Build history of the part. All positions in model axes, mm. Round coordinates to 2 decimals unless told otherwise and drop trailing zeros. Write each loop counter-clockwise with the first axis right and the second up, starting at its lowest first coordinate (ties: lowest second). Pieces come first, ordered by that corner, then holes. Notation, with made-up numbers: (31.25, -10.5) - (47.25, -10.5) arc R25 cw to (47.25, 25.5) - close; hole circle Ø6 at (67, 70). An arc over 180 degrees is marked (long way). Write each question's results on one line, items separated by ' | '.
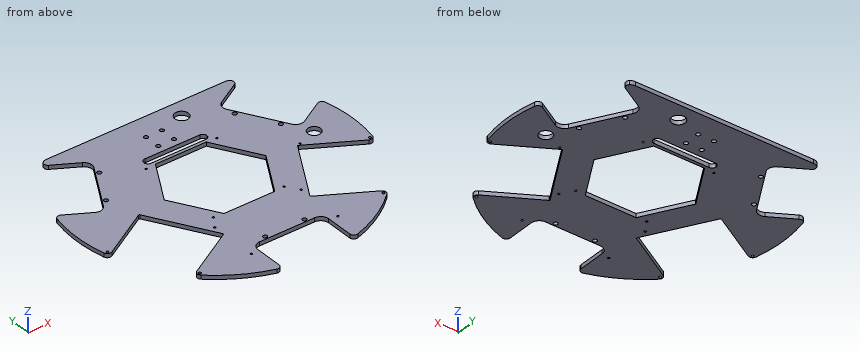
from build123d import *

# Parameters (mm, degrees)
SKETCH_1_R                   = 175
EXTRUDE_1_DEPTH              = 5
CUT_EXTRUDE_1_DEPTH          = 248.53787589
CUT_EXTRUDE_2_DEPTH          = 248.53787589
CUT_EXTRUDE_5_DEPTH          = 248.53787589
CUT_EXTRUDE_4_DEPTH          = 248.53787589
HOLE_WIZARD_M5_1_D           = 5.3
FILLET_1_R                   = 1
FILLET_2_R                   = 10
FILLET_3_R                   = 5
PATTERN_CIRCULAR_1_OUTLINE_R = 2.65
PATTERN_CIRCULAR_1_DEPTH     = 5
HOLE_WIZARD_M5_2_D           = 5.3
SKETCH_15_R                  = 8.55
CUT_EXTRUDE_3_DEPTH          = 243.280431899
MIRROR_1_DEPTH               = 5
SKETCH_18_W                  = 80
SKETCH_18_H                  = 10
CUT_EXTRUDE_6_DEPTH          = 243.280431899
FILLET_4_R                   = 5
M4X0_7_3_D                   = 3.3
SKETCH_33_R                  = 8.05
CUT_EXTRUDE_7_DEPTH          = 243.280431899
M3X0_5_2_D                   = 2.5
M3X0_5_3_D                   = 2.5
FILLET_5_R                   = 10


with BuildPart() as part:
    # 草圖1 → 填料-伸長1 (new body)
    with BuildSketch(Plane.XY):
        Circle(SKETCH_1_R)
    extrude(amount=EXTRUDE_1_DEPTH)

    # 草圖6 → 除料-伸長1 (cut, through all)
    with BuildSketch(Plane.XY.offset(5)):
        with BuildLine():
            Line((-45, -169.115345253), (-45, -118))
            Line((-45, -118), (45, -118))
            Line((45, -118), (45, -169.115345253))
            ThreePointArc((45, -169.115345253), (0, -175), (-45, -169.115345253))
        make_face()
    extrude(amount=-CUT_EXTRUDE_1_DEPTH, mode=Mode.SUBTRACT)

    # 草圖11 → 除料-伸長2 (cut, through all)
    with BuildSketch(Plane.XY.offset(5)):
        Polygon((64.663230149, 0), (32.331615075, 56), (-32.331615075, 56), (-64.663230149, 0), (-32.331615075, -56), (32.331615075, -56), align=None)
    extrude(amount=-CUT_EXTRUDE_2_DEPTH, mode=Mode.SUBTRACT)

    # 草圖17 → 除料-伸長5 (cut, through all)
    with BuildSketch(Plane.XY.offset(5)):
        with BuildLine():
            Line((-169.224997863, -44.585873304), (-100.808990964, -5.085873304))
            Line((-100.808990964, -5.085873304), (-54.808990964, -84.760210452))
            Line((-54.808990964, -84.760210452), (-123.224997863, -124.260210452))
            ThreePointArc((-123.224997863, -124.260210452), (-151.554445662, -87.5), (-169.224997863, -44.585873304))
        make_face()
    extrude(amount=-CUT_EXTRUDE_5_DEPTH, mode=Mode.SUBTRACT)

    # 草圖16 → 除料-伸長4 (cut, through all)
    with BuildSketch(Plane.XY.offset(5)):
        with BuildLine():
            Line((-117.153745139, 130), (117.153745139, 130))
            ThreePointArc((117.153745139, 130), (0, 175), (-117.153745139, 130))
        make_face()
    extrude(amount=-CUT_EXTRUDE_4_DEPTH, mode=Mode.SUBTRACT)

    # M5 餘隙孔1 (through all)
    with Locations(Plane.XY.offset(5)):
        with Locations((25, -114), (-25, -114)):
            Hole(HOLE_WIZARD_M5_1_D / 2)

    # 圓角1
    fillet_1_edges = [part.edges().sort_by_distance(p)[0] for p in [
        (-100.808990964, -5.085873304, 2.5),
        (-54.808990964, -84.760210452, 2.5),
    ]]
    fillet(fillet_1_edges, radius=FILLET_1_R)

    # 圓角2
    fillet_2_edges = [part.edges().sort_by_distance(p)[0] for p in [
        (45, -118, 2.5),
        (-45, -118, 2.5),
    ]]
    fillet(fillet_2_edges, radius=FILLET_2_R)

    # 圓角3
    fillet_3_edges = [part.edges().sort_by_distance(p)[0] for p in [
        (45, -169.115345253, 2.5),
        (-45, -169.115345253, 2.5),
        (-123.224997863, -124.260210452, 2.5),
        (-169.224997863, -44.585873304, 2.5),
    ]]
    fillet(fillet_3_edges, radius=FILLET_3_R)

    # 環狀複製排列1: read off the stored shape, not the designer's step
    # 環狀複製排列1 outline → 環狀複製排列1 (cut)
    with BuildSketch(Plane.XY):
        with BuildLine():
            ThreePointArc((-170.586369053, 39.054970147), (-167.71040421, 42.522591801), (-163.212472795, 42.269240876))
            Line((-163.212472795, 42.269240876), (-133.351251684, 25.02885683))
            ThreePointArc((-133.351251684, 25.02885683), (-125.763061233, 24.029852605), (-119.690997647, 28.689110868))
            Line((-119.690997647, 28.689110868), (-84.690997647, 89.310889132))
            ThreePointArc((-84.690997647, 89.310889132), (-83.691993422, 96.899079583), (-88.351251684, 102.97114317))
            Line((-88.351251684, 102.97114317), (-118.212472795, 120.211527217))
            ThreePointArc((-118.212472795, 120.211527217), (-120.680846839, 123.980174625), (-119.115780818, 128.204644066))
            ThreePointArc((-119.115780818, 128.204644066), (-151.554445662, 87.5), (-170.586369053, 39.054970147))
        make_face()
        with BuildLine():
            ThreePointArc((119.115780818, 128.204644066), (120.680846839, 123.980174625), (118.212472795, 120.211527217))
            Line((118.212472795, 120.211527217), (88.351251684, 102.97114317))
            ThreePointArc((88.351251684, 102.97114317), (83.691993422, 96.899079583), (84.690997647, 89.310889132))
            Line((84.690997647, 89.310889132), (119.690997647, 28.689110868))
            ThreePointArc((119.690997647, 28.689110868), (125.763061233, 24.029852605), (133.351251684, 25.02885683))
            Line((133.351251684, 25.02885683), (163.212472795, 42.269240876))
            ThreePointArc((163.212472795, 42.269240876), (167.71040421, 42.522591801), (170.586369053, 39.054970147))
            ThreePointArc((170.586369053, 39.054970147), (151.554445663, 87.5), (119.115780818, 128.204644066))
        make_face()
        with Locations((86.226896031, 78.650635095)):
            Circle(PATTERN_CIRCULAR_1_OUTLINE_R)
        with Locations((111.226896031, 35.349364905)):
            Circle(PATTERN_CIRCULAR_1_OUTLINE_R)
        with Locations((-111.226896031, 35.349364905)):
            Circle(PATTERN_CIRCULAR_1_OUTLINE_R)
        with Locations((-86.226896031, 78.650635095)):
            Circle(PATTERN_CIRCULAR_1_OUTLINE_R)
    extrude(amount=PATTERN_CIRCULAR_1_DEPTH, mode=Mode.SUBTRACT)

    # M5 餘隙孔2 (through all)
    with Locations(Plane.XY.offset(5)):
        with Locations((10, 100), (-10, 80), (-10, 100), (10, 80)):
            Hole(HOLE_WIZARD_M5_2_D / 2)

    # 草圖15 → 除料-伸長3 (cut, through all)
    with BuildSketch(Plane.XY.offset(5)):
        with Locations((41.5, 108)):
            Circle(SKETCH_15_R)
    extrude(amount=-CUT_EXTRUDE_3_DEPTH, mode=Mode.SUBTRACT)

    # 鏡射1: read off the stored shape, not the designer's step
    # 鏡射1 outline → 鏡射1 (cut)
    with BuildSketch(Plane.XY):
        with BuildLine():
            ThreePointArc((118.323726866, -128.936013823), (151.554445662, -87.5), (170.823726866, -38.003346425))
            ThreePointArc((170.823726866, -38.003346425), (167.955089021, -41.494838656), (163.443048956, -41.247663546))
            Line((163.443048956, -41.247663546), (101.675016368, -5.585873304))
            ThreePointArc((101.675016368, -5.585873304), (100.916197323, -5.485972882), (100.308990964, -5.951898708))
            Line((100.308990964, -5.951898708), (55.308990964, -83.894185049))
            ThreePointArc((55.308990964, -83.894185049), (55.209090541, -84.653004094), (55.675016368, -85.260210452))
            Line((55.675016368, -85.260210452), (117.443048956, -120.922000695))
            ThreePointArc((117.443048956, -120.922000695), (119.913128913, -124.705954459), (118.323726866, -128.936013823))
        make_face()
    extrude(amount=MIRROR_1_DEPTH, mode=Mode.SUBTRACT)

    # 草圖18 → 除料-伸長6 (cut, through all)
    with BuildSketch(Plane.XY.offset(5)):
        with Locations((0, 65)):
            Rectangle(SKETCH_18_W, SKETCH_18_H)
    extrude(amount=-CUT_EXTRUDE_6_DEPTH, mode=Mode.SUBTRACT)

    # 圓角4
    fillet_4_edges = [part.edges().sort_by_distance(p)[0] for p in [
        (40, 70, 2.5),
        (40, 60, 2.5),
        (-40, 60, 2.5),
        (-40, 70, 2.5),
    ]]
    fillet(fillet_4_edges, radius=FILLET_4_R - 0.0001)  # a hair under: the kernel refuses the full size

    # M4x0.7 螺紋孔3 (through all)
    with Locations(Plane.XY.offset(5)):
        with Locations((-116.894870844, -125.224312068), (-166.894870844, -38.621771689)):
            m4x0_7_3 = Hole(M4X0_7_3_D / 2)

    # 鏡射2: M4x0.7 螺紋孔3 across plane
    add(m4x0_7_3.mirror(Plane(origin=(0, 0, 0), x_dir=(0, 0, 1), z_dir=(1, 0, 0))), mode=Mode.SUBTRACT)

    # 草圖33 → 除料-伸長7 (cut, through all)
    with BuildSketch(Plane.XY.offset(5)):
        with Locations((130, 5)):
            Circle(SKETCH_33_R)
    extrude(amount=-CUT_EXTRUDE_7_DEPTH, mode=Mode.SUBTRACT)

    # M3x0.5 螺紋孔2 (through all)
    with Locations(Plane.XY.offset(5)):
        with Locations((55, -130), (55, -70), (-55, -130), (-55, -70)):
            Hole(M3X0_5_2_D / 2)

    # M3x0.5 螺紋孔3 (through all)
    with Locations(Plane.XY.offset(5)):
        with Locations((45, 55), (-45, -55), (-45, 55), (45, -55), (105, -4)):
            Hole(M3X0_5_3_D / 2)

    # 圓角5
    # the kernel refuses this fillet: 10 mm, written as the material it takes off along each edge
    with BuildSketch(Plane(origin=(117.153745139, 130, 14.387351056), x_dir=(-1, 0, 0), z_dir=(0, 0, -1))) as fillet_5_piece_1:
        with BuildLine():
            CenterArc((3.754940423, -10), FILLET_5_R, 90, 34.868690312)
            ThreePointArc((-1.962035679, -1.795355934), (-0.984428411, -0.89395076), (0, 0))
            Line((0, 0), (3.754940423, 0))
        make_face()
    extrude(amount=23.774702113, mode=Mode.SUBTRACT)
    with BuildSketch(Plane(origin=(-117.153745139, 130, 14.387351056), x_dir=(-0.7377488527785091, -0.6750752774498513, 0), z_dir=(0, 0, -1))) as fillet_5_piece_2:
        with BuildLine():
            CenterArc((3.980549786, -9.912355975), FILLET_5_R, 97.591305891, 34.868690312)
            Line((-2.770202989, -2.534867448), (0, 0))
            ThreePointArc((0, 0), (1.329744988, 0.005052135), (2.659489977, 0))
        make_face()
    extrude(amount=23.774702113, mode=Mode.SUBTRACT)


solid = part.part
(1) Flat gauge pins, fed straight in: pin 1 Ø1.5 at (y, z) = (-140.5, 2) entering from -X; pin 2 Ø2 at (y, z) = (37, 3) entering from -X. Where does each tip first touch, or does it go through?
Worked answers:
pin 1: stops at x = -105.33 | pin 2: stops at x = -171.26
(2) Slice it at C-C, the plane z = 2. State how many separate pieces and enclosed holes the cut face has, and give its area (3 significant figures).
Worked answers:
separate pieces: 1 | enclosed holes: 27 | area: 46,500 mm2
(3) Slice it at B-B, the plane y = -105. Write the cut outline in (x, z).
Worked answers:
outline: (-89.87, 0) - (89.87, 0) - (89.87, 5) - (-89.87, 5) - close
(4) Slice it at A-A, the plane x = -76. Write the cut outline in (y, z).
Worked answers:
outline: (-157.64, 0) - (-96.99, 0) - (-96.99, 5) - (-157.64, 5) - close; (-48.06, 0) - (130, 0) - (130, 5) - (-48.06, 5) - close
(5) Drill centre lines: probe 1 along Y at (x, z) = (-32.5, 3.95); probe 2 along Y at (x, z) = (25, 2.6); probe 3 along Y at (x, z) = (-30, 1.35). Where is each one in solid material? Low to high. Write a range as [from, to].
Worked answers:
probe 1: y = [-118, -55.71], [55.71, 60], [70, 130] | probe 2: y = [-118, -116.65], [-111.35, -56], [56, 60], [70, 130] | probe 3: y = [-118, -56], [56, 60], [70, 130]
